The listing builds one solid part. Answer for the finished solid, in the listing's coordinates (mm). A direction names the side the tool comes from. Round coordinates to 2 decimals unless told otherwise and drop trailing zeros. Write each loop counter-clockwise with the first axis right and the second up, starting at its lowest first coordinate (ties: lowest second). Pieces come first, ordered by that corner, then holes. Notation, with made-up numbers: (76.25, 29) - (120.25, 29) arc R26 ccw to (120.25, 67) - close; hole circle Ø9 at (-4, 5.5). An arc over 180 degrees is marked (long way). Return JSON: item names as keys, results as strings. Group by question number.
(1) Section B-B, the plane y = 0 is taken. Give the number of separate pieces and of enclosed holes in the cut face, then the cut area to 3 significant figures.
(2) Determine the mould class of faces 1 (the flat face through (2, 4, -25)), 2 (the cylindrical face through (-2.95, -2.7, -12.32)), 3 (the cylindrical face through (4.38, 8.43, -19.82)) for opening direction X: +X half, -X half, draft (parallel to the pull), parting line (faces both ways), or undercut.
(3) Section A-A, the plane z = -4 is taken. Write down the section's boundary in (x, y), then the cut area to 3 significant figures.
(4) Each of these flat-tipped pins is pushed along its axis until it touches: pin 1 (2 mm diameter, centred on x = -3.5, z = -5.5, fed in from -Y); pin 2 (2 mm diameter, centred on x = -2, z = -10.5, fed in from +Y); pin 3 (1.5 mm diameter, centred on y = 7, z = -14.5, fed in from -X). Where does it stop, or does it pass through?
(5) Section D-D, the plane z = -9 is taken. Write down the section's boundary in (x, y).
(6) Which of the six approach directions +Z, -Z, +X, -X, +Y, -Y give full straight-line access (tool end or side, diameter ignored) to faces 4 (the cylindrical face through (6.53, -0.07, -5.65)), 5 (the cylindrical face through (-0.07, 6.53, -19.35)), 6 (the flat face through (6, 7, -14.5)), 7 (the cylindrical face through (4.38, 8.43, -11.26))?
(7) Find the intervals of material crossed by line 1 along Z through (x, y) = (0, 8); line 2 along Y through (x, z) = (0, -16.25), in increasing order. Write a range as [from, to].
```python
from build123d import *

# Parameters (mm, degrees)
M4X0_7_TAPPED_HOLE1_AT_2_COUNT = 2
M4X0_7_TAPPED_HOLE1_AT_2_PITCH = 17
M4X0_7_TAPPED_HOLE2_AT_2_COUNT = 2
M4X0_7_TAPPED_HOLE2_AT_2_PITCH = 17


with BuildPart() as part:
    # Sketch1 → Revolve3 (revolve)
    with BuildSketch(Plane(origin=(0, 0, 0), x_dir=(1, 0, 0), z_dir=(0, 1, 0))):
        Polygon((4, 0), (9.5, 0), (9.5, 10.5), (9, 10.5), (9, 10.75), (9.5, 10.75), (9.5, 11.75), (9, 11.75), (9, 12), (9.5, 12), (9.5, 13), (9, 13), (9, 13.25), (9.5, 13.25), (9.5, 14.25), (9, 14.25), (9, 14.5), (9.5, 14.5), (9.5, 25), (4, 25), align=None)
    revolve(axis=Axis((0, 0, 0), (0, 0, -1)))

    # Sketch3 → M4x0.7 Tapped Hole1 (revolve, cut)
    with BuildSketch(Plane(origin=(0, 0, -4), x_dir=(0, 0, -1), z_dir=(1, 0, 0))):
        Polygon((0, 0), (0, 11.091420021), (1.65, 10.1), (1.65, 0), align=None)
    m4x0_7_tapped_hole1 = revolve(axis=Axis((0, -6.35, -4), (0, 1, 0)), mode=Mode.SUBTRACT)

    # M4x0.7 Tapped Hole1 at 2: M4x0.7 Tapped Hole1 ×2
    with Locations(*[(0, 0, -i * M4X0_7_TAPPED_HOLE1_AT_2_PITCH) for i in range(1, M4X0_7_TAPPED_HOLE1_AT_2_COUNT)]):
        add(m4x0_7_tapped_hole1, mode=Mode.SUBTRACT)

    # Sketch7 → M4x0.7 Tapped Hole2 (revolve, cut)
    with BuildSketch(Plane(origin=(0, 0, -4), x_dir=(0, 0, 1), z_dir=(0, 1, 0))):
        Polygon((0, 0), (0, 11.091420021), (1.65, 10.1), (1.65, 0), align=None)
    m4x0_7_tapped_hole2 = revolve(axis=Axis((-6.35, 0, -4), (1, 0, 0)), mode=Mode.SUBTRACT)

    # M4x0.7 Tapped Hole2 at 2: M4x0.7 Tapped Hole2 ×2
    with Locations(*[(0, 0, -i * M4X0_7_TAPPED_HOLE2_AT_2_PITCH) for i in range(1, M4X0_7_TAPPED_HOLE2_AT_2_COUNT)]):
        add(m4x0_7_tapped_hole2, mode=Mode.SUBTRACT)


solid = part.part
```
Working result:
{
 "1": {"separate pieces": "4", "enclosed holes": "0", "area": "238 mm^2"},
 "2": {"face 1": "draft", "face 2": "undercut", "face 3": "parting line"},
 "3": {"outline": "(-1.65, 3.64) - (-1.65, 9.36) arc R9.5 ccw (long way) to (9.36, -1.65) - (3.64, -1.65) arc R4 cw (long way) to start; (1.65, 3.64) arc R4 cw to (3.64, 1.65) - (9.36, 1.65) arc R9.5 ccw to (1.65, 9.36) - close", "area": "197 mm^2"},
 "4": {"pin 1": "stops at y = -9.17", "pin 2": "stops at y = 9.45", "pin 3": "stops at x = -7.15"},
 "5": {"outline": "circle Ø19 at (0, 0); hole circle Ø8 at (0, 0)"},
 "6": {"face 4": "+X", "face 5": "+Y", "face 6": "none", "face 7": "+Z, -Z"},
 "7": {"line 1": "z = [-25, -22.65], [-19.35, -5.65], [-2.35, 0]", "line 2": "y = [-9.5, -4], [4, 9.5]"}
}
